```python
from build123d import *

# Parameters (mm, degrees)
SKETCH1_R                   = 17.9
BOSS_EXTRUDE1_DEPTH         = 50
BOSS_EXTRUDE2_START         = 50
SKETCH1_3_R                 = 1.5875
BOSS_EXTRUDE2_DEPTH         = 15
TAP_DRILL_FOR_M3_TAP1_D     = 2.5
TAP_DRILL_FOR_M3_TAP1_DEPTH = 5
TAP_DRILL_FOR_M3_TAP1_TIP   = 0.751075774
SKETCH6_W                   = 2
SKETCH6_H                   = 3


with BuildPart() as part:
    # Sketch1 → Boss-Extrude1 (new body)
    with BuildSketch(Plane.XY):
        Circle(SKETCH1_R)
    extrude(amount=BOSS_EXTRUDE1_DEPTH)

    # Sketch1<3> → Boss-Extrude2 (add)
    with BuildSketch(Plane.XY.offset(BOSS_EXTRUDE2_START)):
        Circle(SKETCH1_3_R)
    extrude(amount=BOSS_EXTRUDE2_DEPTH)

    # Tap Drill for M3 Tap1
    with Locations(Plane.XY.offset(50)):
        with Locations((0, 12.5), (10.825317547, 6.25), (10.825317547, -6.25), (0, -12.5), (-10.825317547, -6.25), (-10.825317547, 6.25)):
            Hole(TAP_DRILL_FOR_M3_TAP1_D / 2, depth=TAP_DRILL_FOR_M3_TAP1_DEPTH)
            with Locations((0, 0, -(TAP_DRILL_FOR_M3_TAP1_DEPTH + TAP_DRILL_FOR_M3_TAP1_TIP / 2))):  # 118° drill point
                Cone(0, TAP_DRILL_FOR_M3_TAP1_D / 2, TAP_DRILL_FOR_M3_TAP1_TIP, mode=Mode.SUBTRACT)

    # Sketch6 → Cut-Revolve1 (revolve, cut)
    with BuildSketch(Plane(origin=(0, 0, 0), x_dir=(0, 0, -1), z_dir=(1, 0, 0))):
        with Locations((-47, 16.4)):
            Rectangle(SKETCH6_W, SKETCH6_H)
        with Locations((-43, 16.4)):
            Rectangle(SKETCH6_W, SKETCH6_H)
        with Locations((-39, 16.4)):
            Rectangle(SKETCH6_W, SKETCH6_H)
        with Locations((-35, 16.4)):
            Rectangle(SKETCH6_W, SKETCH6_H)
        with Locations((-31, 16.4)):
            Rectangle(SKETCH6_W, SKETCH6_H)
        with Locations((-27, 16.4)):
            Rectangle(SKETCH6_W, SKETCH6_H)
        with Locations((-23, 16.4)):
            Rectangle(SKETCH6_W, SKETCH6_H)
        with Locations((-19, 16.4)):
            Rectangle(SKETCH6_W, SKETCH6_H)
        with Locations((-15, 16.4)):
            Rectangle(SKETCH6_W, SKETCH6_H)
        with Locations((-11, 16.4)):
            Rectangle(SKETCH6_W, SKETCH6_H)
        with Locations((-7, 16.4)):
            Rectangle(SKETCH6_W, SKETCH6_H)
        with Locations((-3, 16.4)):
            Rectangle(SKETCH6_W, SKETCH6_H)
    revolve(axis=Axis((0, 0, -3.25), (0, 0, 1)), mode=Mode.SUBTRACT)


solid = part.part
```
Work out the finished part from the listing and answer in its coordinate system (mm). A direction names the side the tool comes from. Give positions to 0.01 mm unless a question says otherwise; leave off trailing zeros. Order: outer loops, then holes, each group sorted by start corner. A loop starts at its lowest first (then second) coordinate and runs counter-clockwise, first axis right, second up. Notation, with made-up numbers: M 49,-16 L 77,-16 A23 cw 77,17 Z; hole C 25.5,60.25 d3. An arc over 180 degrees is marked long. Return JSON: item names as keys, results as strings.
1) Each of these flat-tipped pins is pushed along its axis until it touches: pin 1 (5 mm diameter, centred on x = 7.5, z = 46, fed in from +Y); pin 2 (8 mm diameter, centred on y = -9, z = 30.5, fed in from -X); pin 3 (10 mm diameter, centred on y = 6.5, z = 34, fed in from +X). Where does it stop, or does it pass through?
Resolved:
{"pin 1": "y = 17.19", "pin 2": "x = -17.18", "pin 3": "x = 17.84"}
2) A tool of negligible diameter and unlimited length cuts with its end or side. For faces 1 (the cylindrical face through (10.25, 5.14, 47.46)), 2 (the flat face through (-15, 4, 16)), 3 (the cylindrical face through (17.073, 5.377, 12.986)), from which of +Z, -Z, +X, -X, +Y, -Y can it reach the whole face along a straight path? Write none if from no direction.
Resolved:
{"face 1": "+Z", "face 2": "none", "face 3": "+Z, -Z"}
3) Section B-B, the plane z = 11 is taken. Write down the section's boundary in (x, y).
Resolved:
{"outline": "C 0,0 d29.8"}
4) Section A-A, the plane z = 58 is taken. Write down the section's boundary in (x, y) (1 decimal), plus the area to 3 significant figures.
Resolved:
{"outline": "C 0,0 d3.2", "area": "7.92 mm^2"}
5) Straight lines are drawn through the part: line 1 along Y through (x, z) = (0, 46.4); line 2 along X through (y, z) = (-6.25, 48.05); line 3 along X through (y, z) = (6, 47). For each, find the intervals that lie inside material, in ascending order. Write a range as [from, to].
Resolved:
{"line 1": "[-14.9, -13.75], [-11.25, 11.25], [13.75, 14.9]", "line 2": "[-16.77, -12.08], [-9.58, 9.58], [12.08, 16.77]", "line 3": "[-13.64, -12.05], [-9.6, 9.6], [12.05, 13.64]"}
6) For a pull along Z with two mould halves and no side action, classify faces 4 (the flat face through (4, 0, 50)), 5 (the cylindrical face through (17.073, 5.377, 36.986)), 6 (the flat face through (-15, 4, 36)) as +Z half, -Z half, draft (parallel to the pull), parting line (faces both ways), or undercut.
Resolved:
{"face 4": "+Z half", "face 5": "draft", "face 6": "undercut"}
